Work out the finished part from the listing and answer in its coordinate system (mm). Give positions to 0.01 mm unless a question says otherwise; leave off trailing zeros. Order: outer loops, then holes, each group sorted by start corner. A loop starts at its lowest first (then second) coordinate and runs counter-clockwise, first axis right, second up. Notation, with made-up numbers: (-4.5, 11) - (4.5, 11) arc R18 cw to (4.5, 35) - close; hole circle Ø10 at (67, 19). An arc over 180 degrees is marked (long way). Return JSON: item names as keys, results as strings. Group by question number.
from build123d import *

# Parameters (mm, degrees)
EXTRUDE1_DEPTH = 0.35
FILLET1_R      = 0.37


with BuildPart() as part:
    # Sketch1 → Extrude1 (new body, symmetric)
    with BuildSketch(Plane(origin=(0, 0, 0), x_dir=(0, 0, -1), z_dir=(1, 0, 0))):
        with BuildLine():
            Line((0.048866738, 2.799573546), (0.060647112, 3.474470741))
            ThreePointArc((0.060647112, 3.474470741), (0.747324681, 4.137587561), (0.084207861, 4.824265129))
            Line((0.084207861, 4.824265129), (0.095988235, 5.499162323))
            ThreePointArc((0.095988235, 5.499162323), (0.91428004, 5.423476008), (1.712160583, 5.226710834))
            Line((1.712160583, 5.226710834), (2.304187375, 2.852221062))
            ThreePointArc((2.304187375, 2.852221062), (0, -4.1), (-2.304187375, 2.852221062))
            Line((-2.304187375, 2.852221062), (-1.712160583, 5.226710834))
            ThreePointArc((-1.712160583, 5.226710834), (-0.91428004, 5.423476008), (-0.095988235, 5.499162323))
            Line((-0.095988235, 5.499162323), (-0.084207861, 4.824265129))
            ThreePointArc((-0.084207861, 4.824265129), (-0.747324681, 4.137587561), (-0.060647112, 3.474470741))
            Line((-0.060647112, 3.474470741), (-0.048866738, 2.799573546))
            ThreePointArc((-0.048866738, 2.799573546), (0, -2.8), (0.048866738, 2.799573546))
        make_face()
    extrude(amount=EXTRUDE1_DEPTH, both=True)

    # Fillet1
    fillet1_edges = [part.edges().sort_by_distance(p)[0] for p in [
        (0, 5.226710834, -1.712160583),
        (0, 2.852221062, -2.304187375),
        (0, 2.852221062, 2.304187375),
        (0, 5.226710834, 1.712160583),
    ]]
    fillet(fillet1_edges, radius=FILLET1_R)


solid = part.part
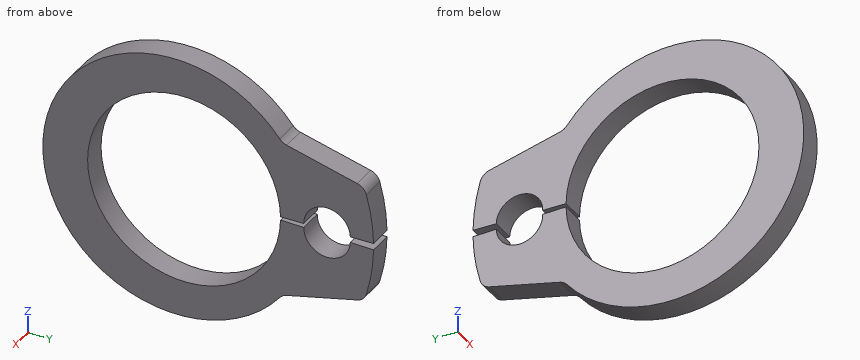
1. The part is cut by section C-C (y = 4). Give the vertices of the cut face in (x, z), and give its area (3 significant figures).
2. The part is cut by section D-D (y = 0). Give the vertices of the cut face in (x, z), and give its area (3 significant figures).
3. Consider probe 1 along Y at (x, z) = (-0.1, 0.5) (3 decimals); probe 2 along Y at (x, z) = (-0.1, 0.25); probe 3 along Z at (x, y) = (0, -2.5). Determine where each line is inside the solid, lowest interval first. Write a range as from..to.
4. The part is cut by section B-B (z = 0.5). Give the vertices of the cut face in (x, y) (3 decimals).
5. The part is cut by section A-A (x = -0.25). Give the vertices of the cut face in (y, z) (3 decimals).
Answers:
{
 "1": {"outline": "(-0.35, -2.02) - (0.35, -2.02) - (0.35, -0.73) - (-0.35, -0.73) - close; (-0.35, 0.73) - (0.35, 0.73) - (0.35, 2.02) - (-0.35, 2.02) - close", "area": "1.80 mm^2"},
 "2": {"outline": "(-0.35, -3.85) - (0.35, -3.85) - (0.35, -2.8) - (-0.35, -2.8) - close; (-0.35, 2.8) - (0.35, 2.8) - (0.35, 3.85) - (-0.35, 3.85) - close", "area": "1.47 mm^2"},
 "3": {"probe 1": "y = -4.067..-2.755, 2.755..3.627, 4.672..5.477", "probe 2": "y = -4.09..-2.79, 2.79..3.5, 4.8..5.49", "probe 3": "z = -3.13..-1.26, 1.26..3.13"},
 "4": {"outline": "(-0.35, -4.067) - (0.35, -4.067) - (0.35, -2.755) - (-0.35, -2.755) - close; (-0.35, 2.755) - (0.35, 2.755) - (0.35, 3.627) - (-0.35, 3.627) - close; (-0.35, 4.672) - (0.35, 4.672) - (0.35, 5.477) - (-0.35, 5.477) - close"},
 "5": {"outline": "(2.777, -2.402) arc R0.37 cw to (2.977, -2.273) - (5.024, -1.763) arc R0.37 ccw to (5.29, -1.505) arc R5.5 ccw to (5.499, -0.096) - (4.824, -0.084) arc R0.675 cw to (3.474, -0.061) - (2.8, -0.049) arc R2.8 cw (long way) to (2.8, 0.049) - (3.474, 0.061) arc R0.675 cw to (4.824, 0.084) - (5.499, 0.096) arc R5.5 ccw to (5.29, 1.505) arc R0.37 ccw to (5.024, 1.763) - (2.977, 2.273) arc R0.37 cw to (2.777, 2.402) arc R3.858 ccw (long way) to start"}
}
